Autodesk Inventor part; units mm, degrees
ref_plane "YZ Plane" through (0, 0, 0) normal (1, 0, 0) x (0, 1, 0)
ref_plane "XZ Plane" through (0, 0, 0) normal (0, 1, 0) x (-1, 0, 0)
ref_plane "XY Plane" through (0, 0, 0) normal (0, 0, 1) x (1, 0, 0)
sketch "Sketch1" plane through (0, 0, 0) normal (0, 0, 1) x (1, 0, 0)
  circle A0 centre (0, 0) radius 3
  dimension "d0" = 6
extrude "Extrusion1" add sketch "Sketch1" along normal mid plane 5.5
fillet "Fillet1" radius 0.2 1 edges at (-3, 0, 2.75)
fillet "Fillet1" radius 0.05 1 edges at (-3, 0, -2.75)
sketch "Sketch2" plane through (0, 0, -2.75) normal (0, 0, -1) x (-1, 0, 0)
  line L0 (1.25, -1.25) -> (-1.25, -1.25)
  line L1 (-1.25, -1.25) -> (-1.25, 1.25)
  line L2 (-1.25, 1.25) -> (1.25, 1.25)
  line L3 (1.25, 1.25) -> (1.25, -1.25)
  line L4 (1.25, -1.25) -> (-1.25, 1.25) construction
  line L5 (-1.25, -1.25) -> (1.25, 1.25) construction
  point P0 (0, 0)
  dimension "d5" = 2.5
extrude "Extrusion2" cut sketch "Sketch2" against normal blind 2.8
sketch "Sketch3" plane through (0, 0, -2.75) normal (0, 0, -1) x (-1, 0, 0)
  circle A0 centre (0, 0) radius 3
  line L0 (-0.9, -3) -> (0.9, -3)
  line L1 (0.9, -3) -> (0.9, 3)
  line L2 (0.9, 3) -> (-0.9, 3)
  line L3 (-0.9, 3) -> (-0.9, -3)
  point P0 (0, 3)
  dimension "d8" = 1.8
extrude "Extrusion3" cut sketch "Sketch3" against normal blind 2 contours L1 A0 L3 | A0 L2 L1 | L1 L0 A0 | A0 L3 L2 | L0 L3 A0
properties part number "48-0077" material "ABS Plastic"
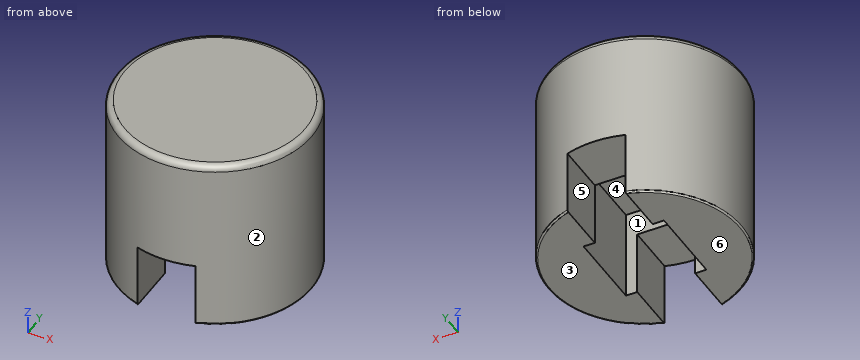
Verification items for the finished model (mm, model axes). Face numbers are marked on the shaded views. A direction names the side the tool comes from. Give positions to 0.01 mm unless a question says otherwise; leave off trailing zeros. Order: outer loops, then holes, each group sorted by start corner. A loop starts at its lowest first (then second) coordinate and runs counter-clockwise, first axis right, second up. Notation, with made-up numbers: M 71.5,76.5 L 101.5,76.5 A15 ccw 101.5,87.5 Z; hole C 30,8.25 d7. An arc over 180 degrees is marked long. Answer in a Markdown table with one row per item. Add a question column.
Item 1: Mould release check, pull along X, two halves, no side actions. Record for the marked faces 1, 2 and 3: released by +X, released by -X, zero draft, split by the parting line, or undercut.
Item 2: Scan lines: probe 1 along Z at (x, y) = (-1, 1); probe 2 along Y at (x, z) = (0.75, -0.55); probe 3 along X at (y, z) = (1, -2.15). Record each from-to range of solid material in increasing order. Write a range as from..to.
Item 3: Section check C-C, the plane y = 0. Enter the section's corners in (x, z).
Item 4: Section check A-A, the plane z = -0.9. Enter the section's corners in (x, y).
Item 5: Section check B-B, the plane x = 0. Enter the section's corners in (y, z).
Item 6: Gauge pin test, flat ends, axial feed: pin 1 (1.3 mm diameter, centred on y = -1.5, z = -1.5, fed in from +X); pin 2 (0.5 mm diameter, centred on x = 0, y = 2, fed in from -Z); pin 3 (1.3 mm diameter, centred on y = -2, z = -1.5, fed in from -X). Record the tip position at first contact, or that the pin passes through.
Item 7: Tool access check on the marked faces 4, 5 and 6. Record the directions out of +Z, -Z, +X, -X, +Y, -Y that give a thin tool (end or side, any length) a straight path to the whole face; none if there is none.
Item 8: Section check D-D, the plane z = 2.05. Enter the section's corners in (x, y), and give its area (3 significant figures).
Filled sheet:
| question | item | result |
|---|---|---|
| 1 | face 1 | undercut |
| 1 | face 2 | split by the parting line |
| 1 | face 3 | zero draft |
| 2 | probe 1 | z = 0.05..2.75 |
| 2 | probe 2 | y = -2.9..-1.25, 1.25..2.9 |
| 2 | probe 3 | x = -2.83..-1.25, 1.25..2.83 |
| 3 | outline | M -3,-2.7 A0.05 ccw -2.95,-2.75 L -1.25,-2.75 L -1.25,0.05 L 1.25,0.05 L 1.25,-2.75 L 2.95,-2.75 A0.05 ccw 3,-2.7 L 3,2.55 A0.2 ccw 2.8,2.75 L -2.8,2.75 A0.2 ccw -3,2.55 Z |
| 4 | outline | M -1.25,-1.25 L -1.25,1.25 L -0.9,1.25 L -0.9,2.86 A3 ccw -0.9,-2.86 L -0.9,-1.25 Z; M 0.9,-2.86 A3 ccw 0.9,2.86 L 0.9,1.25 L 1.25,1.25 L 1.25,-1.25 L 0.9,-1.25 Z |
| 5 | outline | M -3,-0.75 L -1.25,-0.75 L -1.25,0.05 L 1.25,0.05 L 1.25,-0.75 L 3,-0.75 L 3,2.55 A0.2 ccw 2.8,2.75 L -2.8,2.75 A0.2 ccw -3,2.55 Z |
| 6 | pin 1 | stops at x = 2.88 |
| 6 | pin 2 | stops at z = -0.75 |
| 6 | pin 3 | stops at x = -2.68 |
| 7 | face 4 | -Z |
| 7 | face 5 | -Z, +Y, -Y |
| 7 | face 6 | -Z, +X, -X, +Y, -Y |
| 8 | outline | C 0,0 d6 |
| 8 | area | 28.3 mm^2 |
